Geometry: final body of the model. Coordinates: model frame, mm. A direction names the side the tool comes from. Round coordinates to 2 decimals unless told otherwise and drop trailing zeros. Write each loop counter-clockwise with the first axis right and the second up, starting at its lowest first coordinate (ties: lowest second). Pieces come first, ordered by that corner, then holes. Notation, with made-up numbers: (8.5, 52) -> (52.5, 52) arc R22 ccw to (52.5, 72) -> close; hole circle Ø2 at (17, -16.75). An arc over 180 degrees is marked (long way). Use one line per item in the form item = value. Start each with the question number.
1. Cut plane B-B, the plane y = 1.75. State how many separate pieces and enclosed holes the cut face has, plus the area to 3 significant figures.
2. Cut plane A-A, the plane x = 2.5. Return the cut outline in (y, z), plus the area to 3 significant figures.
3. Pin query (flat end, axial travel): pin 1 Ø2.5 at (x, y) = (2.5, 3) entering from -Z; pin 2 Ø1.2 at (y, z) = (4, -11) entering from -X; pin 3 Ø0.9 at (y, z) = (3.5, -11) entering from +X. Return the tip coordinate at first contact, or that it passes through.
4. Line query: L1, parallel to X at y = 4.9, z = 9; L2, parallel to Z at x = 107.5, y = 1.9; L3, parallel to X at y = 1.9, z = -10. Output: solid intervals per line, ascending.
5. Reachability of faces 1 (the face through (54, 0.602, 2)), 2 (the face through (54, 3, -9.863)), 3 (the face through (2, 3, -9.863)) from +Z, -Z, +X, -X, +Y, -Y: full face, straight path, thin tool, end or side. Return the list, or none.
6. Draft query along Z for faces 4 (the face through (78.09, 3.14, -4.22)), 5 (the face through (105, 3, 16)), 6 (the face through (107, 3, -9.863)). Return one class per face: pulls with the +Z half, pulls with the -Z half, needs draft (parallel to the pull), parting line crosses it, or undercut.
7. Cut plane C-C, the plane x = 58.5. Return the cut outline in (y, z), plus the area to 3 significant figures.
```python
from build123d import *

# Parameters (mm, degrees)
SKETCH1_W                      = 27
SKETCH1_H                      = 5
BOSS_EXTRUDE1_DEPTH            = 110
M3_TAPPED_HOLE1_AT_2_COUNT     = 2
M3_TAPPED_HOLE1_AT_2_PITCH     = 7
SKETCH6_W                      = 5
SKETCH6_H                      = 2
CUT_EXTRUDE1_DEPTH             = 10
BOSS_EXTRUDE2_DEPTH            = 5
CUT_EXTRUDE3_DEPTH             = 10
CHAMFER1_SIZE                  = 3
CHAMFER1_OF_MIRROR8_SIZE       = 3
F_3_0MM_DOWEL_HOLE1_AT_2_COUNT = 2
F_3_0MM_DOWEL_HOLE1_AT_2_PITCH = 12.5


with BuildPart() as part:
    # Sketch1 → Boss-Extrude1 (new body)
    with BuildSketch(Plane(origin=(0, 0, 0), x_dir=(0, 0, -1), z_dir=(1, 0, 0))):
        with Locations((-3.636889684, 3.101965352)):
            Rectangle(SKETCH1_W, SKETCH1_H)
    extrude(amount=BOSS_EXTRUDE1_DEPTH)

    # Sketch14 → M3 Tapped Hole1 (revolve, cut)
    with BuildSketch(Plane(origin=(26.397029049, 5.601965352, -4.022332737), x_dir=(0, 0, 1), z_dir=(1, 0, 0))):
        Polygon((0, 0), (0, 8.251075774), (1.25, 7.5), (1.25, 6), (1.5, 6), (1.5, 0), align=None)
    m3_tapped_hole1 = revolve(axis=Axis((26.397029049, 11.951965352, -4.022332737), (0, -1, 0)), mode=Mode.SUBTRACT)

    # M3 Tapped Hole1 at 2: M3 Tapped Hole1 ×2
    with Locations(*[(i * M3_TAPPED_HOLE1_AT_2_PITCH, 0, 0) for i in range(1, M3_TAPPED_HOLE1_AT_2_COUNT)]):
        add(m3_tapped_hole1, mode=Mode.SUBTRACT)

    # Mirror3: M3 Tapped Hole1 across plane
    add(m3_tapped_hole1.mirror(Plane(origin=(55, 0, 0), x_dir=(0, 0, 1), z_dir=(1, 0, 0))), mode=Mode.SUBTRACT)

    # Mirror3 copy 1 sketch → Mirror3 copy 1 (revolve, cut)
    with BuildSketch(Plane(origin=(76.602970951, 5.601965352, -4.022332737), x_dir=(0, 0, 1), z_dir=(-1, 0, 0))):
        Polygon((0, 0), (0, -8.251075774), (1.25, -7.5), (1.25, -6), (1.5, -6), (1.5, 0), align=None)
    revolve(axis=Axis((76.602970951, 11.951965352, -4.022332737), (0, 1, 0)), mode=Mode.SUBTRACT)

    # Sketch6 → Cut-Extrude1 (cut)
    with BuildSketch(Plane(origin=(0, 5.601965352, 0), x_dir=(1, 0, 0), z_dir=(0, 1, 0))):
        with Locations((2.5, -16.136889684)):
            Rectangle(SKETCH6_W, SKETCH6_H)
    cut_extrude1 = extrude(amount=-CUT_EXTRUDE1_DEPTH, mode=Mode.SUBTRACT)

    # Mirror4: Cut-Extrude1 across plane
    add(cut_extrude1.mirror(Plane(origin=(55, 0, 0), x_dir=(0, 0, 1), z_dir=(1, 0, 0))), mode=Mode.SUBTRACT)

    # Sketch17 → Boss-Extrude2 (add)
    with BuildSketch(Plane(origin=(0, 5.601965352, 0), x_dir=(1, 0, 0), z_dir=(0, 1, 0))):
        Polygon((105, 9.863110316), (105, 12.863110316), (103.25, 12.863110316), (99.674047562, 12.863110316), (93.200232163, 12.863110316), (93.200232163, 9.863110316), (97.924047562, 9.863110316), align=None)
    boss_extrude2 = extrude(amount=-BOSS_EXTRUDE2_DEPTH)

    # Sketch22 → Cut-Extrude3 (cut)
    with BuildSketch(Plane(origin=(0, 5.601965352, 0), x_dir=(1, 0, 0), z_dir=(0, 1, 0))):
        with BuildLine():
            Line((101.505065332, 12.863110316), (103.305065332, 12.863110316))
            Line((103.305065332, 12.863110316), (103.305065332, 8.863110316))
            ThreePointArc((103.305065332, 8.863110316), (101.505065332, 7.063110316), (99.705065332, 8.863110316))
            Line((99.705065332, 8.863110316), (99.705065332, 12.863110316))
            Line((99.705065332, 12.863110316), (101.505065332, 12.863110316))
        make_face()
    cut_extrude3 = extrude(amount=-CUT_EXTRUDE3_DEPTH, mode=Mode.SUBTRACT)

    # Chamfer1
    chamfer1_edges = [part.edges().sort_by_distance(p)[0] for p in [
        (93.200232163, 3.101965352, -12.863110316),
    ]]
    chamfer(chamfer1_edges, length=CHAMFER1_SIZE - 0.0001)  # a hair under: the kernel refuses the full size

    # Mirror8: Boss-Extrude2, Cut-Extrude3 across plane
    add(boss_extrude2.mirror(Plane.ZY.offset(-55)))
    add(cut_extrude3.mirror(Plane.ZY.offset(-55)), mode=Mode.SUBTRACT)

    # Chamfer1 of Mirror8
    chamfer1_of_mirror8_edges = [part.edges().sort_by_distance(p)[0] for p in [
        (16.799767837, 3.101965352, -12.863110316),
    ]]
    chamfer(chamfer1_of_mirror8_edges, length=CHAMFER1_OF_MIRROR8_SIZE - 0.0001)  # a hair under: the kernel refuses the full size

    # Sketch24 → Ø3.0mm Dowel Hole1 (revolve, cut)
    with BuildSketch(Plane(origin=(107.5, 0.601965352, -3.613110316), x_dir=(0, 0, -1), z_dir=(1, 0, 0))):
        Polygon((0, 0), (0, 20.901290929), (1.5, 20), (1.5, 0), align=None)
    f_3_0mm_dowel_hole1 = revolve(axis=Axis((107.5, -5.748034648, -3.613110316), (0, 1, 0)), mode=Mode.SUBTRACT)

    # Ø3.0mm Dowel Hole1 at 2: Ø3.0mm Dowel Hole1 ×2
    with Locations(*[(0, 0, i * F_3_0MM_DOWEL_HOLE1_AT_2_PITCH) for i in range(1, F_3_0MM_DOWEL_HOLE1_AT_2_COUNT)]):
        add(f_3_0mm_dowel_hole1, mode=Mode.SUBTRACT)

    # Mirror9: Ø3.0mm Dowel Hole1 across plane
    add(f_3_0mm_dowel_hole1.mirror(Plane.ZY.offset(-55)), mode=Mode.SUBTRACT)

    # Mirror9 copy 1 sketch → Mirror9 copy 1 (revolve, cut)
    with BuildSketch(Plane(origin=(2.5, 0.601965352, 8.886889684), x_dir=(0, 0, -1), z_dir=(-1, 0, 0))):
        Polygon((0, 0), (0, -20.901290929), (1.5, -20), (1.5, 0), align=None)
    revolve(axis=Axis((2.5, -5.748034648, 8.886889684), (0, -1, 0)), mode=Mode.SUBTRACT)


solid = part.part
```
Outcome:
q1.separate_pieces = 1
q1.enclosed_holes = 8
q1.area = 2,920 mm^2
q2.outline = (0.6, -9.86) -> (5.6, -9.86) -> (5.6, -5.11) -> (0.6, -5.11) -> close; (0.6, -2.11) -> (5.6, -2.11) -> (5.6, 7.39) -> (0.6, 7.39) -> close; (0.6, 10.39) -> (5.6, 10.39) -> (5.6, 15.14) -> (0.6, 15.14) -> close
q2.area = 95.0 mm^2
q3.pin_1 = -9.86
q3.pin_2 = 5
q3.pin_3 = 105
q4.L1 = 0 to 1, 4 to 106, 109 to 110
q4.L2 = -9.86 to -5.11, -2.11 to 7.39, 10.39 to 15.14
q4.L3 = 5 to 6.69, 10.29 to 16.66, 93.34 to 99.71, 103.31 to 105
q5.face_1 = +Z, -Z, +X, -X, -Y
q5.face_2 = -Z, +Y, -Y
q5.face_3 = -Z, -X, +Y, -Y
q6.face_4 = undercut
q6.face_5 = needs draft
q6.face_6 = pulls with the -Z half
q7.outline = (0.6, -9.86) -> (5.6, -9.86) -> (5.6, 17.14) -> (0.6, 17.14) -> close
q7.area = 135 mm^2
